Could you check a few things on this model? Use its own coordinates, in mm. Give positions to 0.01 mm unless a question says otherwise; leave off trailing zeros. Write each loop counter-clockwise with the first axis right and the second up, starting at its lowest first coordinate (ties: lowest second). Pieces come first, ordered by that corner, then holes. Notation, with made-up numbers: (-21.75, -5.75) - (-11.75, -5.75) arc R24 ccw to (-11.75, 6.25) - close; hole circle Ø9 at (75, 30.5). An arc over 180 degrees is marked (long way). Answer in a Markdown table with one row per item.
from build123d import *

# Parameters (mm, degrees)
F1_DEPTH = 19.05
F2_DEPTH = 3.175
F3_W     = 12.7
F3_H     = 25.4
F4_DEPTH = 3.175


with BuildPart() as f1:
    # F0 (on Right) → F1 (new body)
    with BuildSketch(Plane.YZ):
        with BuildLine():
            ThreePointArc((-6.35, 0), (0, -6.35), (6.35, 0))
            ThreePointArc((6.35, 0), (0, 6.35), (-6.35, 0))
        make_face()
    extrude(amount=F1_DEPTH)

    # F0 (on Right) → F2 (join)
    with BuildSketch(Plane.YZ):
        with BuildLine():
            ThreePointArc((-6.35, 0), (0, -6.35), (6.35, 0))
            ThreePointArc((6.35, 0), (0, 6.35), (-6.35, 0))
        make_face()
        with BuildLine():
            ThreePointArc((-6.35, 0), (0, 6.35), (6.35, 0))
            Line((6.35, 0), (6.35, 25.4))
            Line((6.35, 25.4), (-6.35, 25.4))
            Line((-6.35, 25.4), (-6.35, 0))
        make_face()
    extrude(amount=F2_DEPTH)

    # F3 (on face) → F4 (join)
    with BuildSketch(Plane.YZ.offset(19.05)):
        with Locations((0, 12.7)):
            Rectangle(F3_W, F3_H)
    extrude(amount=-F4_DEPTH)


solid = f1.part
1) Imagine slicing it at C-C (x = 17). List the corners of the cut face in (y, z) for me.
Check values:
| item | result |
|---|---|
| outline | (-6.35, 0) arc R6.35 ccw to (6.35, 0) - (6.35, 25.4) - (-6.35, 25.4) - close |
2) Imagine slicing it at A-A (z = 17). List the corners of the cut face in (x, y) for me (3 decimals), then the cut area to 3 significant figures.
Check values:
| item | result |
|---|---|
| outline | (0, -6.35) - (3.175, -6.35) - (3.175, 6.35) - (0, 6.35) - close; (15.875, -6.35) - (19.05, -6.35) - (19.05, 6.35) - (15.875, 6.35) - close |
| area | 80.6 mm2 |
3) Will these pins go through, and if not, where does the flat tip stop? P1, Ø4, axis at x = 12, y = -3.5, coming from the +Z side; P2, Ø4, axis at x = 12, z = 6, coming from the +Y side.
Check values:
| item | result |
|---|---|
| P1 | stops at z = 6.17 |
| P2 | stops at y = 4.93 |
4) Imagine slicing it at D-D (y = 2). List the corners of the cut face in (x, z) for me (3 decimals).
Check values:
| item | result |
|---|---|
| outline | (0, -6.027) - (19.05, -6.027) - (19.05, 25.4) - (15.875, 25.4) - (15.875, 6.027) - (3.175, 6.027) - (3.175, 25.4) - (0, 25.4) - close |
5) Imagine slicing it at B-B (y = 0). List the corners of the cut face in (x, z) for me (3 decimals).
Check values:
| item | result |
|---|---|
| outline | (0, -6.35) - (19.05, -6.35) - (19.05, 25.4) - (15.875, 25.4) - (15.875, 6.35) - (3.175, 6.35) - (3.175, 25.4) - (0, 25.4) - close |
6) We'd pull the mould along X, two halves only. Please class faces 1 (the face through (2, 0, 25.4)), 2 (the face through (3.175, 0, 16)), 3 (the face through (9.392, 2.93, -5.634)), 4 (the face through (0, 0, 10)): +X half, -X half, draft (parallel to the pull), parting line (faces both ways), or undercut.
Check values:
| item | result |
|---|---|
| face 1 | draft |
| face 2 | undercut |
| face 3 | undercut |
| face 4 | -X half |
7) If I drill on line 1 (X direction, y = -4.25, z = 15) (3 decimals); line 2 (Z direction, x = 14.75, y = -4.25); line 3 (Z direction, x = 3.75, y = -5), over which ranges is the centre line in solid material (lowest first)?
Check values:
| item | result |
|---|---|
| line 1 | x = 0 to 3.175, 15.875 to 19.05 |
| line 2 | z = -4.72 to 4.72 |
| line 3 | z = -3.91 to 3.91 |
